Check sheet for the modelled part. Datum: model origin and axes. Units: mm. Coordinates: 2 decimals unless noted, no trailing zeros. Loops run counter-clockwise (first coordinate to the right, second up) from the corner with the lowest first, then second, coordinate; pieces in that order, holes last. Notation, with made-up numbers: (-28, -14) - (-4, -14) arc R21 ccw to (-4, 18) - close; hole circle Ø3 at (76, 37.5). An arc over 180 degrees is marked (long way). Use a Markdown table: item, result. Add a question column.
1) Sectioned sample at B-B, the plane z = 0.85. State how many separate pieces and enclosed holes the cut face has, then the cut area to 3 significant figures.
2) Sectioned sample at A-A, the plane x = 9. Enter the section's corners in (y, z).
3) Draft check along Y on faces 1 (the cylindrical face through (14.239, 1.625, 0.626)), 2 (the flat face through (9, -2, 1.27)). Enter one of: pulls with the +Y half, pulls with the -Y half, needs draft (parallel to the pull), parting line crosses it, or undercut.
4) Thickness scan on line 1 (X direction, y = 5.5, z = 0.1); line 2 (X direction, y = 3.75, z = 0.75); line 3 (Y direction, x = 31.5, z = 0.75). Record the ranges inside material, lowest first.
from build123d import *

# Parameters (mm, degrees)
SKETCH1_R           = 3.683
BOSS_EXTRUDE1_DEPTH = 1.27


with BuildPart() as part:
    # Sketch1 → Boss-Extrude1 (new body)
    with BuildSketch(Plane.XY):
        with BuildLine():
            Line((-67.928698338, 11.165767897), (-67.928698338, -5.09495887))
            add(Edge.make_bspline(
                [(-67.928698338, -5.09495887), (-65.317150891, -5.357271388), (-59.445047559, -5.93539969), (-50.370544126, -6.763807956), (-40.79988194, -7.532686473), (-31.506289085, -8.137699048), (-22.575311372, -8.541135315), (-14.081486566, -8.712534782), (-8.230455293, -8.660353622), (-5.219485256, -8.571038003), (-4.87655586, -8.560021553)],
                knots=[0.615514615, 0.615514615, 0.615514615, 0.615514615, 0.63604571, 0.661669949, 0.686792378, 0.711149584, 0.734517597, 0.75671861, 0.777596499, 0.780280213, 0.780280213, 0.780280213, 0.780280213], degree=3))
            Line((-4.87655586, -8.560021553), (36.414501662, -8.775595487))
            Line((36.414501662, -8.775595487), (87.214501662, -8.775595487))
            Line((87.214501662, -8.775595487), (87.214501662, 14.846404513))
            Line((87.214501662, 14.846404513), (36.414501662, 14.846404513))
            Line((36.414501662, 14.846404513), (-4.87655586, 14.63083058))
            add(Edge.make_bspline(
                [(-4.87655586, 14.63083058), (-5.219485256, 14.64184703), (-8.230455293, 14.731162649), (-14.081486566, 14.783343809), (-22.575311372, 14.611944341), (-31.506289085, 14.208508075), (-40.79988194, 13.6034955), (-50.370544126, 12.834616983), (-59.445047559, 12.006208717), (-65.317150891, 11.428080415), (-67.928698338, 11.165767897)],
                knots=[0.219719787, 0.219719787, 0.219719787, 0.219719787, 0.222403501, 0.24328139, 0.265482403, 0.288850416, 0.313207622, 0.338330051, 0.36395429, 0.384485385, 0.384485385, 0.384485385, 0.384485385], degree=3))
        make_face()
        with Locations((10.836701662, 3.035404513)):
            Circle(SKETCH1_R, mode=Mode.SUBTRACT)
        with Locations((-27.263298338, 3.035404513)):
            Circle(SKETCH1_R, mode=Mode.SUBTRACT)
    extrude(amount=BOSS_EXTRUDE1_DEPTH)


solid = part.part
Solved:
| question | item | result |
|---|---|---|
| 1 | separate pieces | 1 |
| 1 | enclosed holes | 2 |
| 1 | area | 3,410 mm2 |
| 2 | outline | (-8.63, 0) - (-0.16, 0) - (-0.16, 1.27) - (-8.63, 1.27) - close; (6.23, 0) - (14.7, 0) - (14.7, 1.27) - (6.23, 1.27) - close |
| 3 | face 1 | undercut |
| 3 | face 2 | needs draft |
| 4 | line 1 | x = -67.93 to -30, -24.53 to 8.1, 13.57 to 87.21 |
| 4 | line 2 | x = -67.93 to -30.88, -23.65 to 7.22, 14.45 to 87.21 |
| 4 | line 3 | y = -8.75 to 14.82 |
